For this review, take the finished solid that the model builds, in its own axes (mm). Face numbers are marked on the shaded views. A direction names the side the tool comes from. Coordinates: 2 decimals unless noted, no trailing zeros. Loops run counter-clockwise (first coordinate to the right, second up) from the corner with the lowest first, then second, coordinate; pieces in that order, holes last. Notation, with made-up numbers: M -10.5,24.5 L 20.5,24.5 A4 ccw 20.5,28.5 Z; hole C 6,54 d11. An arc over 180 degrees is marked long. Answer as a JSON object with one key per item and string values. Group by question number.
Item 1: Insertion check: pin 1 (1 mm diameter, centred on x = 1, y = -7.5, fed in from +Z); pin 2 (3 mm diameter, centred on x = 2, y = -18, fed in from -Z); pin 3 (3 mm diameter, centred on y = -23.5, z = -0.5, fed in from +X). Each pin has a flat end and moves straight along its axis. Give the tip position at first contact, or say it passes through.
Item 2: Wall thickness on L1, parallel to Y at x = 0, z = -0.25; L2, parallel to Y at x = 0.45, z = 2.3; L3, parallel to X at y = -53, z = 0.1: over which ranges is each line inside the solid? List them lowest first. Write a range as from..to.
Item 3: Add section B-B (z = 0). State the section outline as (x, y) points.
Item 4: Add section C-C (y = -53). State the section outline as (x, z) points, then the cut area to 3 significant figures.
Item 5: Add section D-D (y = -42.5). State the section outline as (x, z) points.
Item 6: Tool access review of the marked faces 1 and 2: name each direction out of +Z, -Z, +X, -X, +Y, -Y from which nothing blocks a thin tool from reaching the whole face with its end or side.
Item 7: Add section A-A (x = 0). State the section outline as (y, z) points.
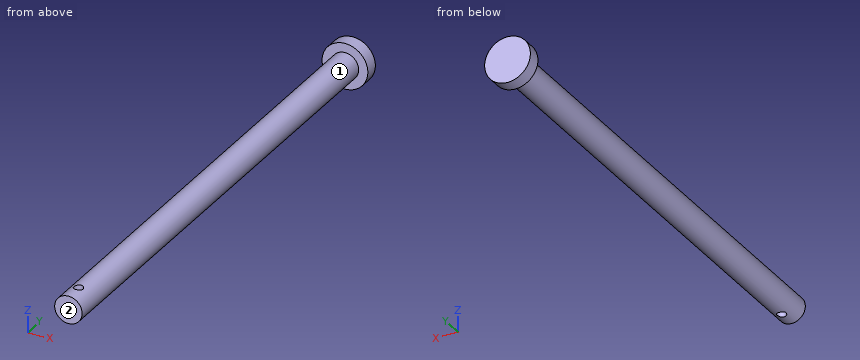
from build123d import *

# Parameters (mm, degrees)
F0_R     = 1.5
F1_DEPTH = 55
F2_R     = 2.5
F2_R_2   = 1.5
F3_DEPTH = 1.5
F4_R     = 0.5
F5_DEPTH = 2.5


with BuildPart() as f1:
    # F0 (on Front) → F1 (new body)
    with BuildSketch(Plane.XZ):
        Circle(F0_R)
    extrude(amount=F1_DEPTH)

    # F2 (on face) → F3 (join)
    with BuildSketch(Plane(origin=(0, 0, 0), x_dir=(-1, 0, 0), z_dir=(0, 1, 0))):
        Circle(F2_R)
        Circle(F2_R_2, mode=Mode.SUBTRACT)
        Circle(F2_R_2)
    extrude(amount=F3_DEPTH)

    # F4 (on Top) → F5 (cut, symmetric)
    with BuildSketch(Plane.XY):
        with Locations((0, -53)):
            Circle(F4_R)
    extrude(amount=F5_DEPTH, both=True, mode=Mode.SUBTRACT)


solid = f1.part
From the geometry:
{
 "1": {"pin 1": "stops at z = 1.41", "pin 2": "stops at z = -1.41", "pin 3": "stops at x = 1.5"},
 "2": {"L1": "y = -55..-53.5, -52.5..1.5", "L2": "y = 0..1.5", "L3": "x = -1.5..-0.5, 0.5..1.5"},
 "3": {"outline": "M -2.5,0 L -1.5,0 L -1.5,-55 L 1.5,-55 L 1.5,0 L 2.5,0 L 2.5,1.5 L -2.5,1.5 Z; hole C 0,-53 d1"},
 "4": {"outline": "M -0.5,-1.41 L -0.5,1.41 A1.5 ccw Z; M 0.5,-1.41 A1.5 ccw 0.5,1.41 Z", "area": "4.13 mm²"},
 "5": {"outline": "C 0,0 d3"},
 "6": {"face 1": "-Y", "face 2": "+Z, -Z, +X, -X, -Y"},
 "7": {"outline": "M -55,-1.5 L -53.5,-1.5 L -53.5,1.5 L -55,1.5 Z; M -52.5,-1.5 L 0,-1.5 L 0,-2.5 L 1.5,-2.5 L 1.5,2.5 L 0,2.5 L 0,1.5 L -52.5,1.5 Z"}
}
